Part model, mm, in its own coordinate system. A direction names the side the tool comes from. Coordinates: 2 decimals unless noted, no trailing zeros. Loops run counter-clockwise (first coordinate to the right, second up) from the corner with the lowest first, then second, coordinate; pieces in that order, holes last. Notation, with made-up numbers: (-8.75, 53.5) - (13.25, 53.5) arc R17 cw to (13.25, 74.5) - close; hole circle Ø8 at (81.5, 14). An arc over 180 degrees is marked (long way). Use a Markdown table: item, result. Add a question column.
1. Band-saw the part on D-D, the plane z = 19. Give the cut face in (x, y).
2. 3-axis set-ups, long thin cutter, end or side, ignore diameter. For faces 1 (the cylindrical face through (26.147, -12.94, 25.222)), 2 (the flat face through (19, -15, 38.1)): which of +Z, -Z, +X, -X, +Y, -Y reach the whole face in a straight line?
3. Drop flat-ended pins along their axis: pin 1 (5 mm diameter, centred on x = 42.5, y = -5, fed in from +Z); pin 2 (1 mm diameter, centred on y = -7.5, z = 11, fed in from +X); pin 3 (12 mm diameter, centred on y = -19, z = 23, fed in from -X). Give the stop position or say it passes through.
4. Band-saw the part on B-B, the plane z = 6. Give the cut face in (x, y), plus the area to 3 significant figures.
5. Band-saw the part on C-C, the plane y = -17.75. Give the cut face in (x, z), plus the area to 3 significant figures.
6. Wall check: probe 1 along Y at (x, z) = (50, 3.5); probe 2 along X at (y, z) = (-16, 9); probe 3 along Z at (x, y) = (45, -21). Give the ranges that are in metal, low to high. Write a range as [from, to].
7. Band-saw the part on A-A, the plane y = -10.25. Give the cut face in (x, z), plus the area to 3 significant figures.
from build123d import *

# Parameters (mm, degrees)
F0_W      = 76.2
F0_H      = 12.7
F1_DEPTH  = 25.4
F3_DEPTH  = 25.4
F4_R      = 6.35
F5_DEPTH  = 50.8
F7_DEPTH  = 25.4
F8_R      = 6.35
F10_DEPTH = 25.4
F12_DEPTH = 25.4
F13_DEPTH = 25.4


# Not quite as in the source:
# - ends of sketch curves that miss each other by under 0.0002 mm in the source are joined


with BuildPart() as f1:
    # F0 (on Front) → F1 (new body)
    with BuildSketch(Plane.XZ):
        with Locations((38.1, 6.35)):
            Rectangle(F0_W, F0_H)
    extrude(amount=F1_DEPTH)

    # F2 (on face) → F3 (cut)
    with BuildSketch(Plane.XY.offset(12.7)):
        with BuildLine():
            ThreePointArc((64.0390142798, 0), (75.4038787349, -12.4300591202), (64.6592453122, -25.4))
            Line((64.6592453122, -25.4), (76.2, -25.4))
            Line((76.2, -25.4), (76.2, 0))
            Line((76.2, 0), (64.0390142798, 0))
        make_face()
    extrude(amount=-F3_DEPTH, mode=Mode.SUBTRACT)

    # F4 (on face) → F5 (cut)
    with BuildSketch(Plane.XY.offset(12.7)):
        with BuildLine():
            ThreePointArc((12.0300554493, -25.4), (3.4859185716, -21.4578724796), (-1.23091e-05, -12.717681963))
            Line((-1.23091e-05, -12.717681963), (0, -25.4))
            Line((0, -25.4), (12.0300554493, -25.4))
        make_face()
        with Locations((12.6999876909, -12.717681963)):
            Circle(F4_R)
    extrude(amount=-F5_DEPTH, mode=Mode.SUBTRACT)

    # F6 (on face) → F7 (cut)
    with BuildSketch(Plane.XY.offset(12.7)):
        with BuildLine():
            ThreePointArc((0, -12.735363926), (3.4749459355, -3.9839181288), (12.0067364357, 0))
            Line((12.0067364357, 0), (0, 0))
            Line((0, 0), (0, -12.735363926))
        make_face()
    extrude(amount=-F7_DEPTH, mode=Mode.SUBTRACT)

    # F8 (on face) → F10 (join)
    with BuildSketch(Plane.XY.offset(12.7)):
        with BuildLine():
            Line((12.0300554493, -25.4), (16.5153164417, -25.4))
            ThreePointArc((16.5153164417, -25.4), (26.1494098267, -12.7), (16.5153164417, 0))
            Line((16.5153164417, 0), (12.0067364357, 0))
            ThreePointArc((12.0067364357, 0), (3.4749459355, -3.9839181288), (0, -12.735363926))
            ThreePointArc((0, -12.735363926), (3.4920052044, -21.4642846479), (12.0300554493, -25.4))
        make_face()
        with Locations((12.6999876909, -12.717681963)):
            Circle(F8_R, mode=Mode.SUBTRACT)
    extrude(amount=F10_DEPTH)

    # F11 (on face) → F12 (cut)
    with BuildSketch(Plane.XY.offset(12.7)):
        with BuildLine():
            Line((39.0294717837, -19.0474465489), (58.5869699212, -19.0474465489))
            ThreePointArc((58.5869699212, -19.0474465489), (52.4176695499, -12.6100109835), (58.7669298396, -6.3500000008))
            Line((58.7669298396, -6.3500000008), (38.9130622506, -6.3503190341))
            ThreePointArc((38.9130622506, -6.3503190341), (43.361986302, -8.2324331506), (45.1994098267, -12.7))
            ThreePointArc((45.1994098267, -12.7), (43.4027543902, -17.126008731), (39.0294717837, -19.0474465489))
        make_face()
        with BuildLine():
            Line((38.6693478697, -19.0474465489), (39.0294717837, -19.0474465489))
            ThreePointArc((39.0294717837, -19.0474465489), (43.4027543902, -17.126008731), (45.1994098267, -12.7))
            ThreePointArc((45.1994098267, -12.7), (43.361986302, -8.2324331506), (38.9130622506, -6.3503190341))
            ThreePointArc((38.9130622506, -6.3503190341), (38.8493077881, -6.3500000008), (38.7855533359, -6.350321083))
            ThreePointArc((38.7855533359, -6.350321083), (32.4996757514, -12.6418865466), (38.6693478697, -19.0474465489))
        make_face()
    extrude(amount=-F12_DEPTH, mode=Mode.SUBTRACT)

    # F9 (on face) → F13 (cut)
    with BuildSketch(Plane.XY.offset(12.7)):
        with BuildLine():
            Line((38.9130622506, -6.3503190341), (38.7855533359, -6.350321083))
            ThreePointArc((38.7855533359, -6.350321083), (32.4994908094, -12.7320698283), (38.8496921889, -19.0499999937))
            ThreePointArc((38.8496921889, -19.0499999937), (43.3396377163, -17.1900282293), (45.1994098267, -12.7))
            ThreePointArc((45.1994098267, -12.7), (43.361986302, -8.2324331506), (38.9130622506, -6.3503190341))
        make_face()
        with BuildLine():
            ThreePointArc((45.1994098267, -12.7), (43.3396377163, -17.1900282293), (38.8496921889, -19.0499999937))
            Line((38.8496921889, -19.0499999937), (58.6612614637, -19.0491190428))
            ThreePointArc((58.6612614637, -19.0491190428), (52.4172516966, -12.6471639759), (58.7669298396, -6.3500000008))
            Line((58.7669298396, -6.3500000008), (38.9130622506, -6.3503190341))
            ThreePointArc((38.9130622506, -6.3503190341), (43.361986302, -8.2324331506), (45.1994098267, -12.7))
        make_face()
        with BuildLine():
            Line((58.8733669384, -19.0491096112), (58.6612614637, -19.0491190428))
            ThreePointArc((58.6612614637, -19.0491190428), (58.7673142404, -19.0499999937), (58.8733669384, -19.0491096112))
        make_face()
        with BuildLine():
            ThreePointArc((58.7669298396, -6.3500000008), (52.4172516966, -12.6471639759), (58.6612614637, -19.0491190428))
            Line((58.6612614637, -19.0491190428), (58.8733669384, -19.0491096112))
            ThreePointArc((58.8733669384, -19.0491096112), (63.294598975, -17.1523742188), (65.1170318782, -12.7))
            ThreePointArc((65.1170318782, -12.7), (63.2571238625, -8.2098358635), (58.7669298396, -6.3500000008))
        make_face()
    extrude(amount=-F13_DEPTH, mode=Mode.SUBTRACT)


solid = f1.part
Geometry check:
| question | item | result |
|---|---|---|
| 1 | outline | (0, -12.74) arc R12.7 ccw to (12.03, -25.4) - (16.52, -25.4) arc R13.19 ccw to (16.52, 0) - (12.01, 0) arc R12.76 ccw to start; hole circle Ø12.7 at (12.7, -12.72) |
| 2 | face 1 | +Z, +X |
| 2 | face 2 | +Z, +X, -X, +Y, -Y |
| 3 | pin 1 | stops at z = 12.7 |
| 3 | pin 2 | stops at x = 74.5 |
| 3 | pin 3 | stops at x = 0 |
| 4 | outline | (0, -12.74) arc R12.7 ccw to (12.03, -25.4) - (64.66, -25.4) arc R12.83 ccw to (64.04, 0) - (12.01, 0) arc R12.76 ccw to start; hole circle Ø12.7 at (12.7, -12.72); hole (38.85, -19.05) - (58.66, -19.05) arc R6.35 ccw (long way) to (58.77, -6.35) - (38.91, -6.35) arc R6.35 ccw (long way) to start |
| 4 | area | 1,270 mm^2 |
| 5 | outline | (1.04, 0) - (8.83, 0) - (8.83, 38.1) - (1.04, 38.1) - close; (16.57, 0) - (35, 0) - (35, 12.7) - (25.14, 12.7) - (25.14, 38.1) - (16.57, 38.1) - close; (62.62, 0) - (74.39, 0) - (74.39, 12.7) - (62.62, 12.7) - close |
| 5 | area | 898 mm^2 |
| 6 | probe 1 | y = [-25.4, -19.05], [-6.35, 0] |
| 6 | probe 2 | x = [0.43, 7.26], [18.14, 33.42], [64.19, 74.99] |
| 6 | probe 3 | z = [0, 12.7] |
| 7 | outline | (0.24, 0) - (6.85, 0) - (6.85, 38.1) - (0.24, 38.1) - close; (18.55, 0) - (32.99, 0) - (32.99, 12.7) - (25.92, 12.7) - (25.92, 38.1) - (18.55, 38.1) - close; (64.63, 0) - (75.16, 0) - (75.16, 12.7) - (64.63, 12.7) - close |
| 7 | area | 756 mm^2 |
